Build history of the part. All positions in model axes, mm. Give positions to 0.01 mm unless a question says otherwise; leave off trailing zeros. Order: outer loops, then holes, each group sorted by start corner. A loop starts at its lowest first (then second) coordinate and runs counter-clockwise, first axis right, second up. Notation, with made-up numbers: (73.25, 11) - (81.25, 11) arc R29 cw to (81.25, 46) - close; hole circle Ø4 at (86.5, 31). An arc over 180 degrees is marked (long way). Answer in a Markdown table with one row per item.
```python
from build123d import *

# Parameters (mm, degrees)
SKETCH1_R           = 4.6
SKETCH1_R_2         = 1.5
BOSS_EXTRUDE1_DEPTH = 10.2
BOSS_EXTRUDE2_DEPTH = 8
SKETCH3_R           = 3.6
CUT_EXTRUDE1_DEPTH  = 5
SKETCH4_R           = 1.5
BOSS_EXTRUDE3_DEPTH = 0.6
SKETCH5_R           = 1.5
BOSS_EXTRUDE4_DEPTH = 4
FILLET1_R           = 2


with BuildPart() as part:
    # Sketch1 → Boss-Extrude1 (new body)
    with BuildSketch(Plane.XY):
        with BuildLine():
            Line((-118.85, 7.5), (-2.75, 7.5))
            Line((-2.75, 7.5), (-2.75, 3.5))
            ThreePointArc((-2.75, 3.5), (1.25, -0.5), (5.25, 3.5))
            Line((5.25, 3.5), (5.25, 7.5))
            Line((5.25, 7.5), (97.25, 7.5))
            Line((97.25, 7.5), (97.25, 3.5))
            ThreePointArc((97.25, 3.5), (101.25, -0.5), (105.25, 3.5))
            Line((105.25, 3.5), (105.25, 7.5))
            Line((105.25, 7.5), (119.25, 7.5))
            Line((119.25, 7.5), (124.013139721, 15.75))
            ThreePointArc((124.013139721, 15.75), (131.526279442, 17.763139721), (133.539419162, 10.25))
            Line((133.539419162, 10.25), (125.312177826, -4))
            ThreePointArc((125.312177826, -4), (122.75, -6.562177826), (119.25, -7.5))
            Line((119.25, -7.5), (-118.85, -7.5))
            ThreePointArc((-118.85, -7.5), (-124.082590181, -5.332590181), (-126.25, -0.1))
            Line((-126.25, -0.1), (-126.25, 0.1))
            ThreePointArc((-126.25, 0.1), (-124.082590181, 5.332590181), (-118.85, 7.5))
        make_face()
        with Locations((-118.75, 0)):
            Circle(SKETCH1_R, mode=Mode.SUBTRACT)
        with Locations((128.776279442, 13)):
            Circle(SKETCH1_R_2, mode=Mode.SUBTRACT)
    extrude(amount=BOSS_EXTRUDE1_DEPTH)

    # Sketch2 → Boss-Extrude2 (add)
    with BuildSketch(Plane(origin=(0, 0, 0), x_dir=(-1, 0, 0), z_dir=(0, 0, -1))):
        with BuildLine():
            Line((-105.25, 3.5), (-105.25, 7.5))
            Line((-105.25, 7.5), (-97.25, 7.5))
            Line((-97.25, 7.5), (-97.25, 3.5))
            ThreePointArc((-97.25, 3.5), (-101.25, -0.5), (-105.25, 3.5))
        make_face()
        with BuildLine():
            Line((-5.25, 3.5), (-5.25, 7.5))
            Line((-5.25, 7.5), (2.75, 7.5))
            Line((2.75, 7.5), (2.75, 3.5))
            ThreePointArc((2.75, 3.5), (-1.25, -0.5), (-5.25, 3.5))
        make_face()
    extrude(amount=-BOSS_EXTRUDE2_DEPTH)

    # Sketch3 → Cut-Extrude1 (cut)
    with BuildSketch(Plane(origin=(0, 0, 0), x_dir=(-1, 0, 0), z_dir=(0, 0, -1))):
        with Locations((-128.776279442, 13)):
            Circle(SKETCH3_R)
    extrude(amount=-CUT_EXTRUDE1_DEPTH, mode=Mode.SUBTRACT)

    # Sketch4 → Boss-Extrude3 (add)
    with BuildSketch(Plane(origin=(0, 0, 5), x_dir=(-1, 0, 0), z_dir=(0, 0, -1))):
        with Locations((-128.776279442, 13)):
            Circle(SKETCH4_R)
    extrude(amount=-BOSS_EXTRUDE3_DEPTH)

    # Sketch5 → Boss-Extrude4 (add)
    with BuildSketch(Plane.XY.offset(10.2)):
        with BuildLine():
            Line((-88.75, 7.5), (-88.75, -7.5))
            Line((-88.75, -7.5), (119.25, -7.5))
            ThreePointArc((119.25, -7.5), (122.75, -6.562177826), (125.312177826, -4))
            Line((125.312177826, -4), (133.539419162, 10.25))
            ThreePointArc((133.539419162, 10.25), (131.526279442, 17.763139721), (124.013139721, 15.75))
            Line((124.013139721, 15.75), (119.25, 7.5))
            Line((119.25, 7.5), (105.25, 7.5))
            Line((105.25, 7.5), (105.25, 3.5))
            ThreePointArc((105.25, 3.5), (101.25, -0.5), (97.25, 3.5))
            Line((97.25, 3.5), (97.25, 7.5))
            Line((97.25, 7.5), (5.25, 7.5))
            Line((5.25, 7.5), (5.25, 3.5))
            ThreePointArc((5.25, 3.5), (1.25, -0.5), (-2.75, 3.5))
            Line((-2.75, 3.5), (-2.75, 7.5))
            Line((-2.75, 7.5), (-88.75, 7.5))
        make_face()
        with Locations(Location((128.776279442, 13, 0), (0, 0, 180))):
            Circle(SKETCH5_R, mode=Mode.SUBTRACT)
    extrude(amount=BOSS_EXTRUDE4_DEPTH)

    # Fillet1
    fillet1_edges = [part.edges().sort_by_distance(p)[0] for p in [
        (-88.75, 7.5, 12.2),
        (-88.75, -7.5, 12.2),
    ]]
    fillet(fillet1_edges, radius=FILLET1_R)


solid = part.part
```
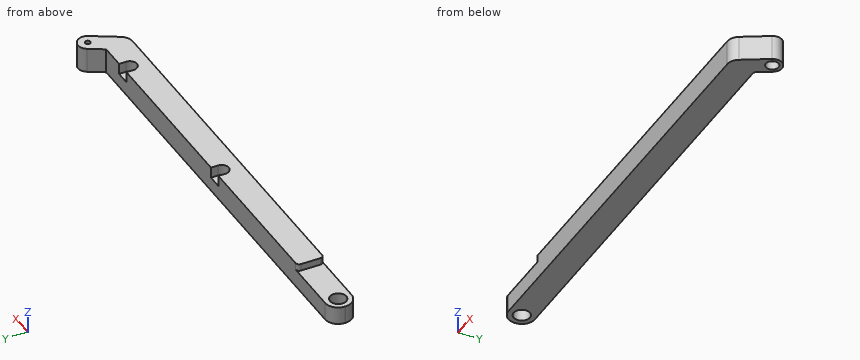
1. Drop flat-ended pins along their axis: P1, Ø2, axis at y = 6.5, z = 10.5, coming from the +X side; P2, Ø1.2, axis at y = 6, z = 11.5, coming from the -X side; P3, Ø1.8, axis at x = 128.78, y = 13, coming from the -Z side. Give the stop position or say it passes through.
Check result:
| item | result |
|---|---|
| P1 | stops at x = 131.95 |
| P2 | stops at x = -88.75 |
| P3 | stops at z = 5 |
2. Cut at A-A on x = 1.25. Write the cut outline in (y, z), and give its area (3 significant figures).
Check result:
| item | result |
|---|---|
| outline | (-7.5, 0) - (7.5, 0) - (7.5, 8) - (-0.5, 8) - (-0.5, 14.2) - (-7.5, 14.2) - close |
| area | 163 mm² |
3. Probe line 1 (Y direction, x = -118.75, z = 7.25); line 2 (Y direction, x = 0.5, z = 4.5); line 3 (X direction, y = 1.75, z = 4). List the from-to ranges inside material, lowest first.
Check result:
| item | result |
|---|---|
| line 1 | y = -7.5 to -4.6, 4.6 to 7.5 |
| line 2 | y = -7.5 to 7.5 |
| line 3 | x = -126.06 to -123, -114.5 to 128.63 |
4. Cut at B-B on x = 42. Write the cut outline in (y, z).
Check result:
| item | result |
|---|---|
| outline | (-7.5, 0) - (7.5, 0) - (7.5, 14.2) - (-7.5, 14.2) - close |
